Verification items for this drawing (mm, ordinates from the low corner). A direction names the side the tool comes from. Round coordinates to 2 decimals unless told otherwise and drop trailing zeros. Loops run counter-clockwise (first coordinate to the right, second up) from the corner with the lowest first, then second, coordinate; pieces in that order, holes last. Notation, with made-up numbers: (15.25, 20.25) - (37.25, 20.25) arc R18 cw to (37.25, 54.25) - close; hole circle Ø10 at (-34.75, 6.25). An arc over 180 degrees is marked (long way). Put each result on its own line as item: value.
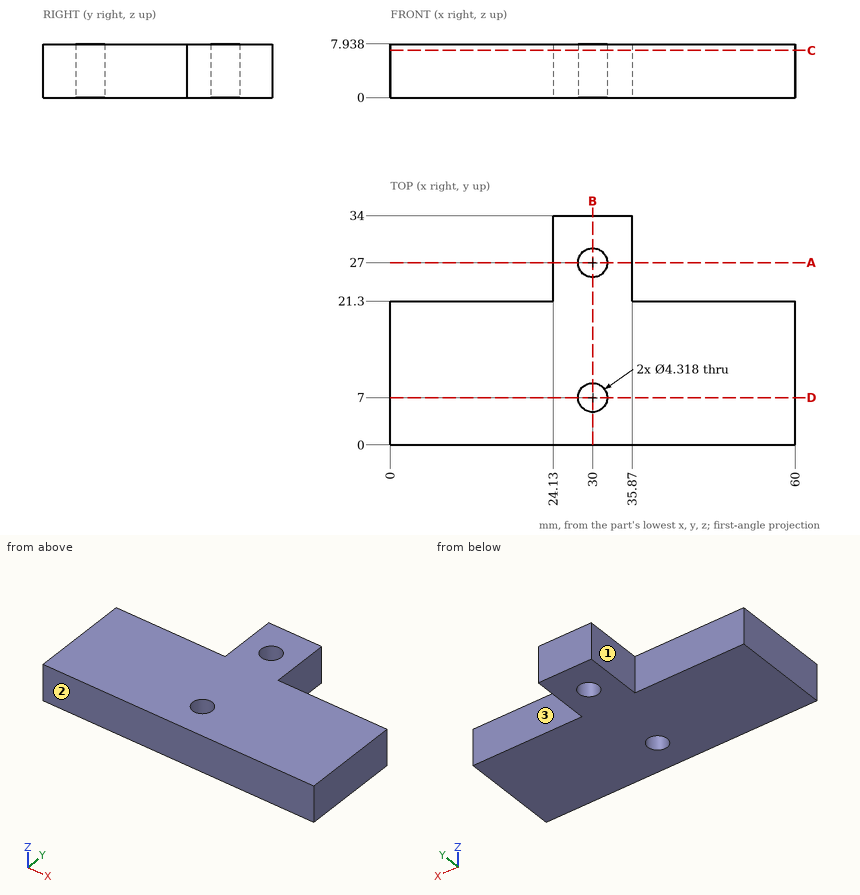
Item 1: Tool access check on the marked faces 1, 2 and 3. Record the directions out of +Z, -Z, +X, -X, +Y, -Y that give a thin tool (end or side, any length) a straight path to the whole face; none if there is none.
Filled sheet:
face 1: +Z, -Z, -X, +Y
face 2: +Z, -Z, +X, -X, -Y
face 3: +Z, -Z, +X, +Y
Item 2: Section check A-A on y = 27. Enter the section's corners in (x, z).
Filled sheet:
outline: (24.13, 0) - (27.84, 0) - (27.84, 7.94) - (24.13, 7.94) - close; (32.16, 0) - (35.87, 0) - (35.87, 7.94) - (32.16, 7.94) - close
Item 3: Thickness scan on line 1 (Y direction, x = 30, z = 6.25); line 2 (Y direction, x = 21, z = 1.5); line 3 (X direction, y = 24.5, z = 2.5). Record the ranges inside material, lowest first. Write a range as from..to.
Filled sheet:
line 1: 0..4.84, 9.16..24.84, 29.16..34
line 2: 0..21.3
line 3: 24.13..35.87
Item 4: Section check D-D on y = 7. Enter the section's corners in (x, z).
Filled sheet:
outline: (0, 0) - (27.84, 0) - (27.84, 7.94) - (0, 7.94) - close; (32.16, 0) - (60, 0) - (60, 7.94) - (32.16, 7.94) - close
Item 5: Section check B-B on x = 30. Enter the section's corners in (y, z).
Filled sheet:
outline: (0, 0) - (4.84, 0) - (4.84, 7.94) - (0, 7.94) - close; (9.16, 0) - (24.84, 0) - (24.84, 7.94) - (9.16, 7.94) - close; (29.16, 0) - (34, 0) - (34, 7.94) - (29.16, 7.94) - close
Item 6: Go/stop test with flat-tipped pins: pin 1 (5.5 mm diameter, centred on x = 30, y = 27, fed in from +Z); pin 2 (4 mm diameter, centred on x = 43.5, z = 5.5, fed in from +Y); pin 3 (2.5 mm diameter, centred on x = 30, y = 7, fed in from -Z). Record where each tip stops, or that it passes through.
Filled sheet:
pin 1: z = 7.94
pin 2: y = 21.3
pin 3: through
Item 7: Section check C-C on z = 7. Enter the section's corners in (x, y), then the cut area to 3 significant figures.
Filled sheet:
outline: (0, 0) - (60, 0) - (60, 21.3) - (35.87, 21.3) - (35.87, 34) - (24.13, 34) - (24.13, 21.3) - (0, 21.3) - close; hole circle Ø4.32 at (30, 7); hole circle Ø4.32 at (30, 27)
area: 1,400 mm²
